Here's the drawing with two shaded views (mm, measured from the low corner). I have some questions. Coordinates: 2 decimals unless noted, no trailing zeros. Order: outer loops, then holes, each group sorted by start corner. A loop starts at its lowest first (then second) coordinate and runs counter-clockwise, first axis right, second up. Notation, with made-up numbers: (46, 9) -> (98, 9) arc R27 ccw to (98, 45) -> close; hole circle Ø7 at (76, 53.25). An arc over 180 degrees is marked (long way). Answer as a JSON object with one key per item and string values. Group by question number.
(1) I want a section at C-C, the plane z = 3. List the corners of the cut face in (x, y) for me (1 decimal).
(2) I need wall thicknesses on line 1 (X direction, y = 51, z = 4) (1 decimal); line 2 (X direction, y = 7.5, z = 5.75) (1 decimal); line 3 (X direction, y = 20, z = 1.75) (1 decimal). Which ranges of each line are inside material? Lowest first, please.
(3) I want a section at A-A, the plane x = 13.2. List the corners of the cut face in (y, z) for me.
(4) I want a section at D-D, the plane x = 51. List the corners of the cut face in (y, z) for me, plus the area to 3 significant figures.
(5) I want a section at B-B, the plane x = 41. List the corners of the cut face in (y, z) for me (1 decimal).
(6) For pin 1 (13.5 mm diameter, centred on x = 56.37, y = 13.2, fed in from -Z); pin 2 (4 mm diameter, centred on y = 41.5, z = 5, fed in from -X) (1 decimal); pin 3 (3 mm diameter, centred on x = 62, z = 1.5, fed in from -Y); pin 4 (3 mm diameter, centred on y = 31.5, z = 5, fed in from -X), each with a flat end and sliding along its axis, tell me the tip position at first contact or that it passes through.
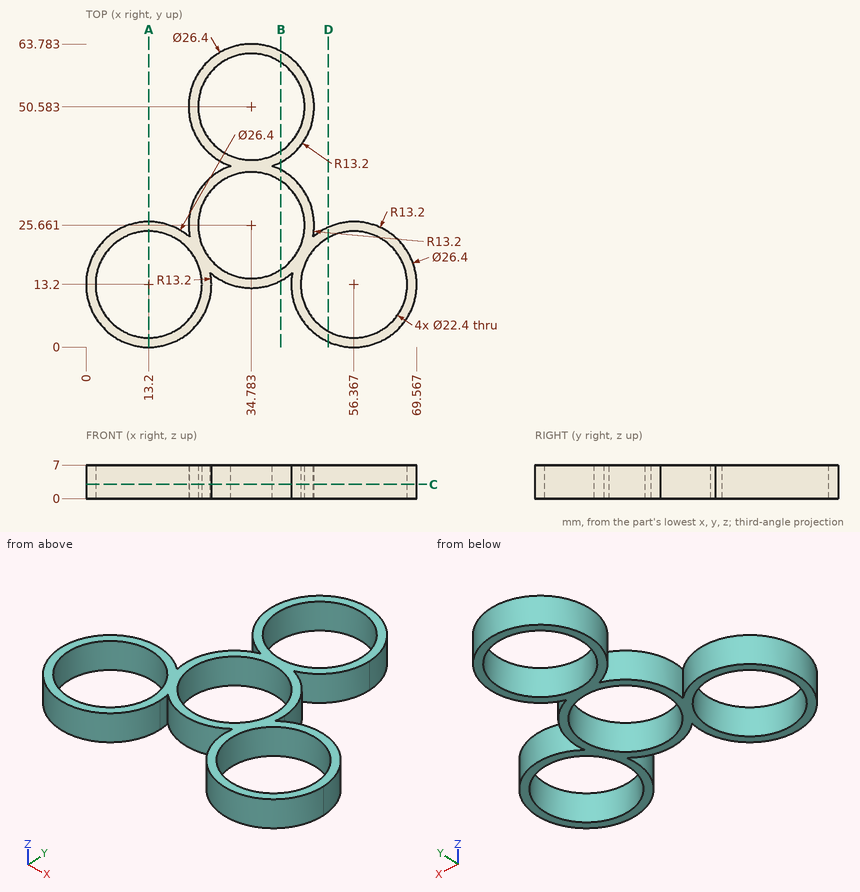
Computed values:
{
 "1": {"outline": "(21.8, 23.2) arc R13.2 ccw (long way) to (26.2, 15.7) arc R13.2 ccw to (43.4, 15.7) arc R13.2 ccw (long way) to (47.8, 23.2) arc R13.2 ccw to (39.1, 38.1) arc R13.2 ccw (long way) to (30.4, 38.1) arc R13.2 ccw to start; hole circle Ø22.4 at (13.2, 13.2); hole circle Ø22.4 at (34.8, 25.7); hole circle Ø22.4 at (34.8, 50.6); hole circle Ø22.4 at (56.4, 13.2)"},
 "2": {"line 1": "x = 21.6 to 23.6, 46 to 48", "line 2": "x = 1.3 to 3.6, 22.8 to 25.1, 44.5 to 46.7, 66 to 68.3", "line 3": "x = 1.9 to 4.3, 22.1 to 25.1, 44.4 to 47.5, 65.3 to 67.7"},
 "3": {"outline": "(0, 0) -> (2, 0) -> (2, 7) -> (0, 7) -> close; (24.4, 0) -> (26.4, 0) -> (26.4, 7) -> (24.4, 7) -> close"},
 "4": {"outline": "(1.14, 0) -> (3.37, 0) -> (3.37, 7) -> (1.14, 7) -> close; (23.03, 0) -> (25.26, 0) -> (25.26, 7) -> (23.03, 7) -> close", "area": "31.2 mm2"},
 "5": {"outline": "(14, 0) -> (16.3, 0) -> (16.3, 7) -> (14, 7) -> close; (35, 0) -> (37.3, 0) -> (37.3, 7) -> (35, 7) -> close; (38.9, 0) -> (41.3, 0) -> (41.3, 7) -> (38.9, 7) -> close; (59.9, 0) -> (62.2, 0) -> (62.2, 7) -> (59.9, 7) -> close"},
 "6": {"pin 1": "passes through", "pin 2": "stops at x = 23.6", "pin 3": "stops at y = 0.66", "pin 4": "stops at x = 22.32"}
}
